Read the model definition and answer for the solid it produces. Units are mm, in the model's axes. A direction names the side the tool comes from. Round coordinates to 2 decimals unless told otherwise and drop trailing zeros. Write each loop counter-clockwise with the first axis right and the second up, starting at its lowest first coordinate (ties: lowest second). Pieces come first, ordered by that corner, then holes. Notation, with made-up numbers: (11.5, 87) -> (41.5, 87) arc R29 ccw to (41.5, 126) -> close; hole circle Ø9 at (30.5, 60). An arc over 180 degrees is marked (long way). Return JSON: item names as keys, results as strings. Group by question number.
(1) Straight lines are drawn through the part: line 1 (X direction, y = -16.5, z = 61.5); line 2 (Z direction, x = -17, y = -14); line 3 (X direction, y = -14, z = 14). For each, find the intervals that lie inside material, in ascending order.
(2) Given pin 1 (6.5 mm diameter, centred on x = 73.62, z = 105.28, fed in from -Y); pin 2 (4.5 mm diameter, centred on x = 67.51, z = 8.48, fed in from -Y), each flat-ended and moving along its own axis, determine where each tip first touches the part or whether it passes through.
(3) A cutting plane is placed at B-B on y = -7.5. Give the vertices of the cut face in (x, z).
(4) For faces 4 (the flat face through (26, -19, -51)), 5 (the cylindrical face through (93.459, -16.972, 81.126)), determine the directions among +Z, -Z, +X, -X, +Y, -Y from which every point of the face is accessible in a straight line to the end or side of a thin tool.
(5) The mould has two halves that part along Z. Classify faces 1 (the flat face through (47, -15, 3)), 2 (the flat face through (106.691, -9, -17)), 3 (the flat face through (26, -9, 160.1)): released by +Z, released by -Z, zero draft, split by the parting line, or undercut.
(6) A cutting plane is placed at A-A on x = 9. Give the vertices of the cut face in (y, z).
(7) A cutting plane is placed at C-C on x = -8.5. Give the vertices of the cut face in (y, z), then the cut area to 3 significant figures.
```python
from build123d import *

# Parameters (mm, degrees)
F0_R     = 70
F0_R_2   = 60
F1_DEPTH = 15
F0_W     = 160
F0_H     = 350
F2_DEPTH = 19
F4_D     = 5


with BuildPart() as f1:
    # F0 (on Front) → F1 (new body)
    with BuildSketch(Plane.XZ):
        with Locations((26.691287, 60.099899)):
            Circle(F0_R)
        with Locations((26.691287, 60.099899)):
            Circle(F0_R_2, mode=Mode.SUBTRACT)
    extrude(amount=F1_DEPTH)

    # F0 (on Front) → F2 (join)
    with BuildSketch(Plane.XZ):
        with Locations((26.691287, -14.900101)):
            Rectangle(F0_W, F0_H)
        with Locations((26.691287, 60.099899)):
            Circle(F0_R, mode=Mode.SUBTRACT)
    extrude(amount=F2_DEPTH)

    # F4 (through all)
    with Locations(Plane.XZ.offset(15)):
        with Locations((-26.138766, 98.351955), (73.61643, 105.279788), (67.508727, 8.484681)):
            Hole(F4_D / 2)


solid = f1.part
```
Checks:
{
 "1": {"line 1": "x = -53.31 to -43.29, 96.68 to 106.69", "line 2": "z = -189.9 to 18.98, 101.22 to 160.1", "line 3": "x = -53.31 to -11.71, 65.09 to 106.69"},
 "2": {"pin 1": "stops at y = -15", "pin 2": "passes through"},
 "3": {"outline": "(-53.31, -189.9) -> (106.69, -189.9) -> (106.69, 160.1) -> (-53.31, 160.1) -> close; hole circle Ø120 at (26.69, 60.1); hole circle Ø5 at (-26.14, 98.35); hole circle Ø5 at (67.51, 8.48); hole circle Ø5 at (73.62, 105.28)"},
 "4": {"face 4": "+Z, -Z, +X, -X, -Y", "face 5": "-Y"},
 "5": {"face 1": "undercut", "face 2": "zero draft", "face 3": "released by +Z"},
 "6": {"outline": "(-19, -189.9) -> (0, -189.9) -> (0, 2.77) -> (-15, 2.77) -> (-15, -7.63) -> (-19, -7.63) -> close; (-19, 127.83) -> (-15, 127.83) -> (-15, 117.43) -> (0, 117.43) -> (0, 160.1) -> (-19, 160.1) -> close"},
 "7": {"outline": "(-19, -189.9) -> (0, -189.9) -> (0, 11.5) -> (-15, 11.5) -> (-15, -0.41) -> (-19, -0.41) -> close; (-19, 120.61) -> (-15, 120.61) -> (-15, 108.7) -> (0, 108.7) -> (0, 160.1) -> (-19, 160.1) -> close", "area": "4,710 mm^2"}
}
